The model under review builds one solid part; all positions refer to its coordinate system, in mm. A direction names the side the tool comes from. Give positions to 0.01 mm unless a question says otherwise; leave off trailing zeros. Loops run counter-clockwise (first coordinate to the right, second up) from the corner with the lowest first, then second, coordinate; pieces in that order, holes last. Notation, with made-up numbers: M 80.25,-26 L 97.25,-26 A32 cw 97.25,9 Z; hole C 21.5,33.25 d9. An arc over 180 degrees is marked long. Write item = value, one per line. Start each with the question number.
1. Wall thickness on line 1 along X through (y, z) = (0, -394); line 2 along Y through (x, z) = (-8.5, -191.5) (3 decimals); line 3 along Z through (x, y) = (-145.5, 29.5): over which ranges is each line inside the solid? List them lowest first. Write a range as from..to.
2. We need section C-C on z = -253. Give the boundary of the cut face in (x, y), then the cut area to 3 significant figures.
3. For faces 4 (the face through (-130.38, 17.12, 76.05)), 5 (the face through (-130.38, 17.12, -372.26)), 6 (the face through (-60.3, 27.4, 150)), list the 3-axis set-ups (+Z, -Z, +X, -X, +Y, -Y) from which the entire face can be reached by the end or side of a thin tool; tool diameter is ignored.
4. Draft analysis for pull direction Z (two halves, no side actions). For faces 1 (the face through (-131.1, -12.6, 0)), 2 (the face through (-7.035, 159.845, -50.7)), 3 (the face through (-30, 127, -637)), state which applies: pulls with the +Z half, pulls with the -Z half, needs draft (parallel to the pull), parting line crosses it, or undercut.
5. We need section A-A on y = 0. Give the boundary of the cut face in (x, z), then the cut area to 3 significant figures.
6. For pin 1 (6 mm diameter, centred on y = 88.5, z = -598, fed in from -X); pin 2 (1 mm diameter, centred on x = 24.5, z = -562.5, fed in from +Y); pin 3 (5 mm diameter, centred on x = -44, z = -707, fed in from -Y), all flat-tipped, find the tip position at first contact; note any pin that passes through.
7. We need section D-D on y = -93.5. Give the boundary of the cut face in (x, z).
from build123d import *

# Parameters (mm, degrees)
SKETCH2_R          = 66
CUT_EXTRUDE1_DEPTH = 984.386495738


with BuildPart() as part:
    # Sketch1 → Revolve1 (revolve)
    with BuildSketch(Plane(origin=(0, 0, 0), x_dir=(0, 0, -1), z_dir=(1, 0, 0)), mode=Mode.PRIVATE) as revolve1_sk:
        Polygon((0, 160), (100, 160), (100, 131.5), (637, 131.5), (637, 130), (807, 130), (807, 0), (-150, 0), (-150, 131.5), (-100, 131.5), (-50, 131.5), (0, 131.5), align=None)
    revolve(revolve1_sk.sketch.rotate(Axis((0, 0, 150), (0, 0, -1)), 180), axis=Axis((0, 0, 150), (0, 0, -1)))

    # Sketch2 → Cut-Extrude1 (cut, through all)
    with BuildSketch(Plane(origin=(0, 0, -807), x_dir=(-1, 0, 0), z_dir=(0, 0, -1))):
        with Locations(Location((0, 0, 0), (0, 0, 90))):
            Circle(SKETCH2_R)
    extrude(amount=-CUT_EXTRUDE1_DEPTH, mode=Mode.SUBTRACT)


solid = part.part
Final values:
q1.line_1 = -131.5..-66, 66..131.5
q1.line_2 = -131.225..-65.45, 65.45..131.225
q1.line_3 = -100..0
q2.outline = C 0,0 d263; hole C 0,0 d132
q2.area = 40,600 mm²
q3.face_4 = +Z
q3.face_5 = -Z
q3.face_6 = +Z, +X, -X, +Y, -Y
q4.face_1 = pulls with the +Z half
q4.face_2 = needs draft
q4.face_3 = pulls with the -Z half
q5.outline = M -160,-100 L -131.5,-100 L -131.5,-637 L -130,-637 L -130,-807 L -66,-807 L -66,150 L -131.5,150 L -131.5,0 L -160,0 Z; M 66,-807 L 130,-807 L 130,-637 L 131.5,-637 L 131.5,-100 L 160,-100 L 160,0 L 131.5,0 L 131.5,150 L 66,150 Z
q5.area = 131,000 mm²
q6.pin_1 = -99.91
q6.pin_2 = 129.29
q6.pin_3 = -123.2
q7.outline = M -129.84,-100 L -92.47,-100 L -92.47,-637 L -90.32,-637 L -90.32,-807 L 90.32,-807 L 90.32,-637 L 92.47,-637 L 92.47,-100 L 129.84,-100 L 129.84,0 L 92.47,0 L 92.47,150 L -92.47,150 L -92.47,0 L -129.84,0 Z
